Input: dimensioned drawing with shaded views. Units: mm. Origin: part minimum x, y, z. Give positions to 0.01 mm unless a question says otherwise; leave off trailing zeros. Order: outer loops, then holes, each group sorted by start corner. A loop starts at its lowest first (then second) coordinate and runs counter-clockwise, first axis right, second up. Notation, with made-up numbers: (36.25, 33) -> (70.25, 33) arc R17 cw to (70.25, 66) -> close; hole circle Ø10 at (39.5, 13.25). An arc over 180 degrees is marked (long way). Use CSV: the item, a comma, the result in double quotes.
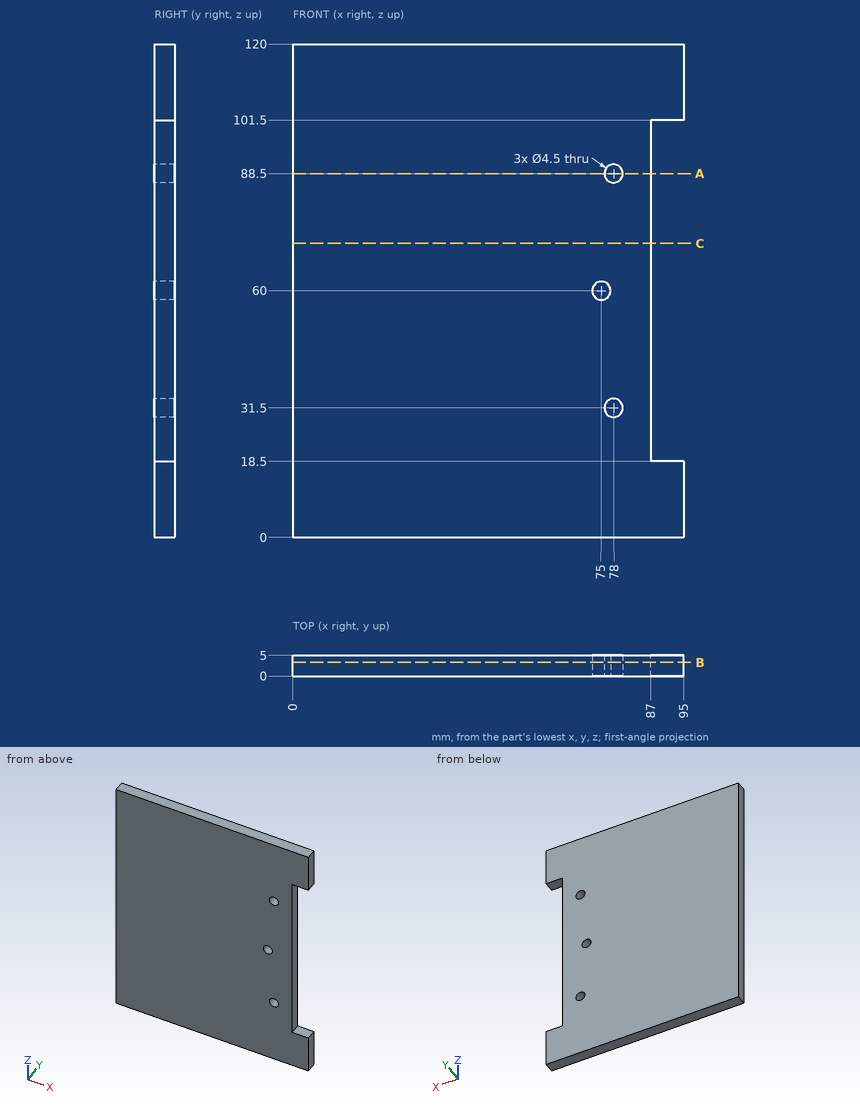
1. Section query B-B on y = 3.3. Return loops of the section in (x, z).
Answer below:
outline,"(0, 0) -> (95, 0) -> (95, 18.5) -> (87, 18.5) -> (87, 101.5) -> (95, 101.5) -> (95, 120) -> (0, 120) -> close; hole circle Ø4.5 at (75, 60); hole circle Ø4.5 at (78, 31.5); hole circle Ø4.5 at (78, 88.5)"
2. Section query C-C on z = 71.5. Return loops of the section in (x, y).
Answer below:
outline,"(0, 0) -> (87, 0) -> (87, 5) -> (0, 5) -> close"
3. Pin query (flat end, axial travel): P1, Ø1.5, axis at x = 91, y = 3, coming from the -Z side; P2, Ø4, axis at x = 75, z = 60, coming from the -Y side; P3, Ø1.5, axis at y = 1.5, z = 72, coming from the +X side. Return the tip coordinate at first contact, or that it passes through.
Answer below:
P1,"stops at z = 0"
P2,"passes through"
P3,"stops at x = 87"
4. Ray query, line 1 along Z through (x, y) = (78, 3.45); line 2 along Z through (x, y) = (75, 3.95); line 3 along X through (y, z) = (2.85, 60). Return the intervals inside material, ascending.
Answer below:
line 1,"z = 0 to 29.25, 33.75 to 86.25, 90.75 to 120"
line 2,"z = 0 to 57.75, 62.25 to 120"
line 3,"x = 0 to 72.75, 77.25 to 87"
5. Section query A-A on z = 88.5. Return loops of the section in (x, y), plus the area to 4 significant figures.
Answer below:
outline,"(0, 0) -> (75.75, 0) -> (75.75, 5) -> (0, 5) -> close; (80.25, 0) -> (87, 0) -> (87, 5) -> (80.25, 5) -> close"
area,"412.5 mm²"
